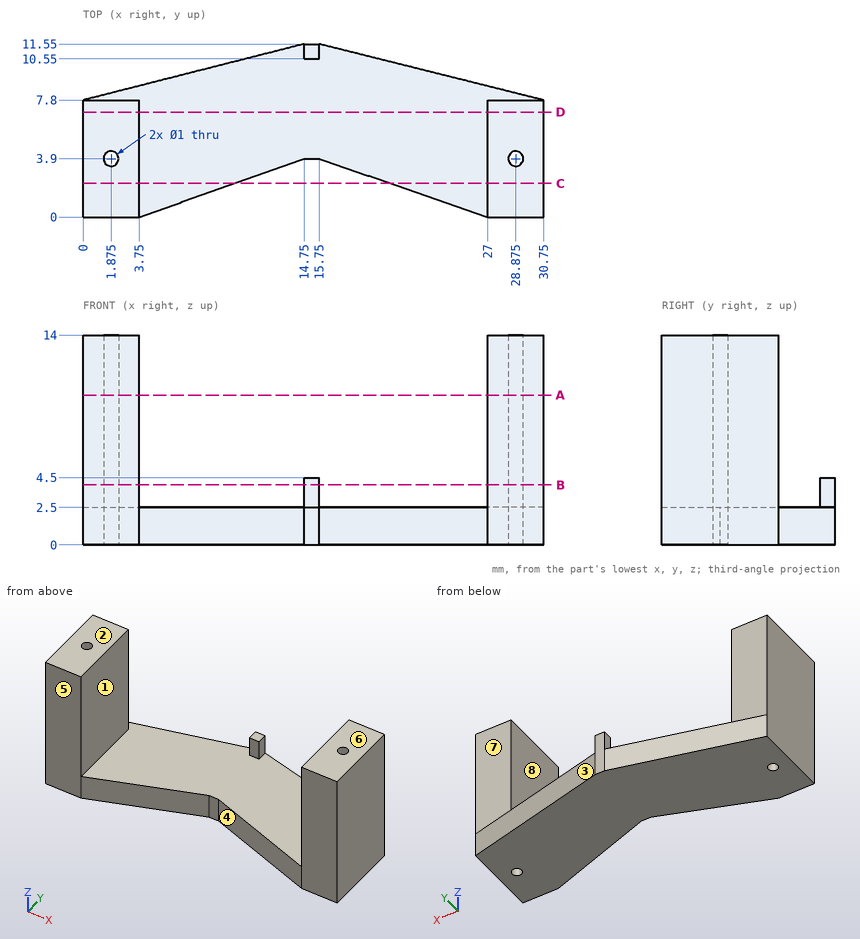
Design review of the part shown in the three views and the two pictorial views. Dimensions are in mm from the part's minimum x, y and z. A direction names the side the tool comes from. Give positions to 0.01 mm unless a question says otherwise; leave off trailing zeros. Loops run counter-clockwise (first coordinate to the right, second up) from the corner with the lowest first, then second, coordinate; pieces in that order, holes last. Notation, with made-up numbers: M 35.25,37 L 52.25,37 A34 cw 52.25,71 Z; hole C -14,64 d10. An arc over 180 degrees is marked long. Put each result on its own line as item: value. Start each with the question number.
(1) Machinability: for the marked faces 4, 5, 6, 7 and 8, which of the approach directions +Z, -Z, +X, -X, +Y, -Y give a long, thin tool a straight path to every point of the face, cutting with its end or side? Answer none if there is none.
(2) Add section D-D, the plane y = 7. Write out the cut boundary in (x, z).
(3) Wall thickness on L1, parallel to X at y = 1.75, z = 3.25; L2, parallel to Z at x = 23, y = 4.5: over which ranges is each line inside the solid? List them lowest first.
(4) Add section C-C, the plane y = 2.25. Write out the cut boundary in (x, z).
(5) Add section B-B, the plane z = 4. Write out the cut boundary in (x, y) (3 decimals).
(6) For pin 1 (1.1 mm diameter, centred on x = 2, z = 10, fed in from +Y); pin 2 (3 mm diameter, centred on y = 9, z = 9, fed in from +X); pin 3 (0.5 mm diameter, centred on y = 11, z = 3.5, fed in from -X); pin 4 (3 mm diameter, centred on x = 7.5, y = 6, fed in from +Z), all flat-tipped, find the tip position at first contact; note any pin that passes through.
(7) The part is to be moulded in two halves that separate along X. For the marked faces 1, 2 and 3, say which applies: +X half, -X half, draft (parallel to the pull), parting line (faces both ways), or undercut.
(8) Add section A-A, the plane z = 10. Write out the cut boundary in (x, y) (3 decimals).
Result:
1. face 4: +Z, -Z, -Y
1. face 5: +Z, -Z, +X, -X, -Y
1. face 6: +Z, +X, -X, +Y, -Y
1. face 7: +Z, +X, -X, +Y
1. face 8: +Z, +Y, -Y
2. outline: M 0,0 L 30.75,0 L 30.75,14 L 27,14 L 27,2.5 L 3.75,2.5 L 3.75,14 L 0,14 Z
3. L1: x = 0 to 3.75, 27 to 30.75
3. L2: z = 0 to 2.5
4. outline: M 0,0 L 10.1,0 L 10.1,2.5 L 3.75,2.5 L 3.75,14 L 0,14 Z; M 20.51,0 L 30.75,0 L 30.75,14 L 27,14 L 27,2.5 L 20.51,2.5 Z
5. outline: M 0,0 L 3.75,0 L 3.75,7.8 L 0,7.8 Z; M 14.75,10.55 L 15.75,10.55 L 15.75,11.55 L 14.75,11.55 Z; M 27,0 L 30.75,0 L 30.75,7.8 L 27,7.8 Z; hole C 1.875,3.9 d1; hole C 28.875,3.9 d1
6. pin 1: stops at y = 7.8
6. pin 2: stops at x = 30.75
6. pin 3: stops at x = 14.75
6. pin 4: stops at z = 2.5
7. face 1: undercut
7. face 2: draft
7. face 3: +X half
8. outline: M 0,0 L 3.75,0 L 3.75,7.8 L 0,7.8 Z; M 27,0 L 30.75,0 L 30.75,7.8 L 27,7.8 Z; hole C 1.875,3.9 d1; hole C 28.875,3.9 d1
